from build123d import *

# Parameters (mm, degrees)
BOSS_EXTRUDE1_DEPTH = 135
SKETCH3_R           = 3.5
CUT_EXTRUDE2_DEPTH  = 10
SKETCH6_W           = 11
SKETCH6_H           = 36
CUT_EXTRUDE3_DEPTH  = 40
SKETCH7_W           = 55
SKETCH7_H           = 16.435142828
BOSS_EXTRUDE2_DEPTH = 35
CUT_EXTRUDE4_DEPTH  = 20
CUT_EXTRUDE5_DEPTH  = 20
SKETCH12_R          = 4.5
CUT_EXTRUDE6_DEPTH  = 20
CUT_EXTRUDE7_DEPTH  = 120
SKETCH14_W          = 10
SKETCH14_H          = 112.990035736
BOSS_EXTRUDE3_DEPTH = 9
SKETCH16_W          = 117.700647477
SKETCH16_H          = 151.246123551
CUT_EXTRUDE11_DEPTH = 166.309899973


with BuildPart() as part:
    # Sketch2 → Boss-Extrude1 (new body)
    with BuildSketch(Plane.XY):
        with BuildLine():
            Line((-7.403081865, 56.261800555), (-7.403081865, -78.738199445))
            ThreePointArc((-7.403081865, -78.738199445), (0.096918135, -86.238199445), (7.596918135, -78.738199445))
            Line((7.596918135, -78.738199445), (7.596918135, 56.261800555))
            ThreePointArc((7.596918135, 56.261800555), (0.096918135, 63.761800555), (-7.403081865, 56.261800555))
        make_face()
    extrude(amount=BOSS_EXTRUDE1_DEPTH)

    # Sketch3 → Cut-Extrude2 (cut)
    with BuildSketch(Plane(origin=(0, 0, 0), x_dir=(-1, 0, 0), z_dir=(0, 0, -1))):
        with Locations((-0.096918135, 54.761800555)):
            Circle(SKETCH3_R)
    extrude(amount=-CUT_EXTRUDE2_DEPTH, mode=Mode.SUBTRACT)

    # Sketch6 → Cut-Extrude3 (cut)
    with BuildSketch(Plane(origin=(0, 0, 0), x_dir=(-1, 0, 0), z_dir=(0, 0, -1))):
        with Locations((-0.096918135, -48.578199445)):
            Rectangle(SKETCH6_W, SKETCH6_H)
    extrude(amount=-CUT_EXTRUDE3_DEPTH, mode=Mode.SUBTRACT)

    # Sketch7 → Boss-Extrude2 (add)
    with BuildSketch(Plane.ZY.offset(7.403081865)):
        with Locations((67.5, -49.750557846)):
            Rectangle(SKETCH7_W, SKETCH7_H)
    extrude(amount=BOSS_EXTRUDE2_DEPTH)

    # Sketch10 → Cut-Extrude4 (cut)
    with BuildSketch(Plane(origin=(0, -41.532986432, 0), x_dir=(1, 0, 0), z_dir=(0, 1, 0))):
        with BuildLine():
            Line((-7.403081865, -40), (-42.403081865, -40))
            Line((-42.403081865, -40), (-42.403081865, -95))
            Line((-42.403081865, -95), (-7.403081865, -95))
            ThreePointArc((-7.403081865, -95), (-33.21161021, -67.5), (-7.403081865, -40))
        make_face()
    extrude(amount=-CUT_EXTRUDE4_DEPTH, mode=Mode.SUBTRACT)

    # Sketch11 → Cut-Extrude5 (cut)
    with BuildSketch(Plane(origin=(0, -41.532986432, 0), x_dir=(1, 0, 0), z_dir=(0, 1, 0))):
        with BuildLine():
            Line((-7.569996139, -52.041059143), (-7.569996139, -82.958940857))
            ThreePointArc((-7.569996139, -82.958940857), (-23.028936996, -67.5), (-7.569996139, -52.041059143))
        make_face()
    extrude(amount=-CUT_EXTRUDE5_DEPTH, mode=Mode.SUBTRACT)

    # Sketch12 → Cut-Extrude6 (cut)
    with BuildSketch(Plane.XY.offset(135)):
        with Locations((0.096918135, 54.761800555)):
            Circle(SKETCH12_R)
    extrude(amount=-CUT_EXTRUDE6_DEPTH, mode=Mode.SUBTRACT)

    # Sketch13 → Cut-Extrude7 (cut)
    with BuildSketch(Plane.XY.offset(135)):
        Polygon((4.403081865, 46.751836291), (-4.403081865, 46.751836291), (-4.403081865, -46.751836291), (-4.403081865, -66.238199445), (4.403081865, -66.238199445), (4.403081865, -46.751836291), align=None)
    extrude(amount=-CUT_EXTRUDE7_DEPTH, mode=Mode.SUBTRACT)

    # Sketch14 → Boss-Extrude3 (add)
    with BuildSketch(Plane.ZY.offset(-4.403081865)):
        with Locations((130, -9.743181577)):
            Rectangle(SKETCH14_W, SKETCH14_H)
    extrude(amount=BOSS_EXTRUDE3_DEPTH)

    # Sketch16 → Cut-Extrude11 (cut, through all)
    with BuildSketch(Plane(origin=(7.596918135, 0, 0), x_dir=(0, 0, -1), z_dir=(1, 0, 0))):
        with Locations((-76.149676262, -11.861261221)):
            Rectangle(SKETCH16_W, SKETCH16_H)
    extrude(amount=-CUT_EXTRUDE11_DEPTH, mode=Mode.SUBTRACT)


solid = part.part
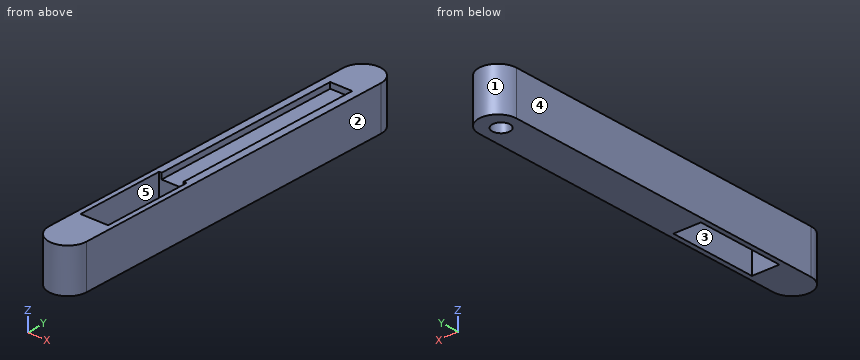
Read the model definition and answer for the solid it produces. Units are mm, in the model's axes. Face numbers are marked on the shaded views. A direction names the side the tool comes from. Give positions to 0.01 mm unless a question says otherwise; leave off trailing zeros. Write each loop counter-clockwise with the first axis right and the second up, starting at its lowest first coordinate (ties: lowest second). Pieces come first, ordered by that corner, then holes. Notation, with made-up numbers: (5, 39.5) - (13, 39.5) arc R35 cw to (13, 74.5) - close; hole circle Ø11 at (38, 81). An arc over 180 degrees is marked (long way). Answer in a Markdown table with one row per item. Add a question column.
Item 1: A tool of negligible diameter and unlimited length cuts with its end or side. For the marked faces 4 and 5, from which of +Z, -Z, +X, -X, +Y, -Y can it reach the whole face along a straight path? Write none if from no direction.
Item 2: Section D-D, the plane y = 8 is taken. Write down the section's boundary in (x, z).
Item 3: Find the intervals of material crossed by L1, parallel to X at y = -34, z = 13; L2, parallel to Y at x = 1.5, z = 3; L3, parallel to Y at x = -2.25, z = 8.75, in increasing order.
Item 4: Section A-A, the plane z = 13.25 is taken. Write down the section's boundary in (x, y).
Item 5: Section C-C, the plane x = 2.25 is taken. Write down the section's boundary in (y, z), and give its area (3 significant figures).
Item 6: Flat-ended cylindrical pins translate along their axes: P1, Ø3.5, axis at x = -1.5, z = 12, coming from the -Y side; P2, Ø4, axis at x = 5.5, z = 12.5, coming from the -Y side; P3, Ø8, axis at x = 5, z = 7, coming from the +Y side. Find the tip coordinate at first contact, or state that the pin passes through.
Item 7: Determine the mould class of the marked faces 1, 2 and 3 for opening direction Y: pulls with the +Y half, pulls with the -Y half, needs draft (parallel to the pull), parting line crosses it, or undercut.
Item 8: Section B-B, the plane y = -52.5 is taken. Write down the section's boundary in (x, z), and give its area (3 significant figures).
Recorded:
| question | item | result |
|---|---|---|
| 1 | face 4 | +Z, -Z, -X, +Y, -Y |
| 1 | face 5 | +Z, -Z |
| 2 | outline | (-7.4, 0) - (7.6, 0) - (7.6, 17.3) - (4.4, 17.3) - (4.4, 15) - (-4.4, 15) - (-4.4, 17.3) - (-7.4, 17.3) - close |
| 3 | L1 | x = -7.4 to -5.4, 5.6 to 7.6 |
| 3 | L2 | y = -86.11 to -66.58, -30.58 to 51.56, 57.97 to 63.63 |
| 3 | L3 | y = -85.86 to -66.58, -30.58 to 52.17, 57.36 to 63.39 |
| 4 | outline | (-7.4, -78.74) arc R7.5 ccw to (7.6, -78.74) - (7.6, 56.26) arc R7.5 ccw to (-7.4, 56.26) - close; hole (-5.4, -66.58) - (5.6, -66.58) - (5.6, -30.58) - (-5.4, -30.58) - close |
| 5 | outline | (-85.92, 0) - (-66.58, 0) - (-66.58, 17.3) - (-85.92, 17.3) - close; (-30.58, 0) - (52, 0) - (52, 10) - (57.52, 10) - (57.52, 0) - (63.45, 0) - (63.45, 17.3) - (46.75, 17.3) - (46.75, 15) - (-30.58, 15) - close |
| 5 | area | 1,730 mm2 |
| 6 | P1 | stops at y = -86.24 |
| 6 | P2 | stops at y = -85.42 |
| 6 | P3 | stops at y = 63.71 |
| 7 | face 1 | pulls with the +Y half |
| 7 | face 2 | needs draft |
| 7 | face 3 | undercut |
| 8 | outline | (-7.4, 0) - (-5.4, 0) - (-5.4, 17.3) - (-7.4, 17.3) - close; (5.6, 0) - (7.6, 0) - (7.6, 17.3) - (5.6, 17.3) - close |
| 8 | area | 69.2 mm2 |
